Build history of the part. All positions in model axes, mm. A direction names the side the tool comes from. Coordinates: 2 decimals unless noted, no trailing zeros. Loops run counter-clockwise (first coordinate to the right, second up) from the corner with the lowest first, then second, coordinate; pieces in that order, holes last.
Item 1: 3-axis set-ups, long thin cutter, end or side, ignore diameter. For faces 4 (the face through (3, 325, -28)), 5 (the face through (206, -5, -25)), 6 (the face through (3, 331, -25)), 7 (the face through (224, -5, -56)): which of +Z, -Z, +X, -X, +Y, -Y reach the whole face in a straight line?
Item 2: Mould opens along X. For faces 1 (the face through (3, -331, -25)), 2 (the face through (-206, -5, -25)), 3 (the face through (3, -325, -28)) say: released by +X, released by -X, zero draft, split by the parting line, or undercut.
Item 3: Flat gauge pins, fed straight in: pin 1 (25 mm diameter, centred on y = -57, z = -19.5, fed in from +X); pin 2 (15 mm diameter, centred on x = 37.5, z = -15, fed in from -Y); pin 3 (15 mm diameter, centred on y = 155.5, z = -23.5, fed in from -X). Where does each tip first touch, or does it go through?
Item 4: Cut at A-A (z = -41). List the corners of the cut face in (x, y), and give its area (3 significant figures).
Item 5: Drill centre lines: line 1 along Y through (x, z) = (-88, -45); line 2 along X through (y, z) = (-148.5, -13.5); line 3 along Y through (x, z) = (74.5, -51). Where is each one in solid material? Low to high.
Item 6: Cut at C-C (y = -205). List the corners of the cut face in (x, z), and give its area (3 significant figures).
Item 7: Cut at B-B (x = 146.5). List the corners of the cut face in (y, z).
Item 8: Cut at D-D (x = 224). List the corners of the cut face in (y, z).
from build123d import *

# Parameters (mm, degrees)
SKETCH054_W            = 400
SKETCH054_H            = 60
PAD003_DEPTH           = 325
SKETCH055_W            = 412
SKETCH055_H            = 50
PAD008_DEPTH           = 331
SKETCH056_W            = 512
SKETCH056_H            = 762
PAD009_DEPTH           = 6
CUT003_PLACEMENT_ANGLE = 180


with BuildPart() as body002:
    # Sketch054 → Pad003 (new body, symmetric)
    with BuildSketch(Plane.XZ):
        with Locations((0, 30)):
            Rectangle(SKETCH054_W, SKETCH054_H)
    extrude(amount=PAD003_DEPTH, both=True)


with BuildPart() as cut003:
    # Sketch055 → Pad008 (new body, symmetric)
    with BuildSketch(Plane.XZ):
        with Locations((0, 25)):
            Rectangle(SKETCH055_W, SKETCH055_H)
    extrude(amount=PAD008_DEPTH, both=True)

    # Sketch056 (on Face3 of Pad008) → Pad009 (join)
    with BuildSketch(Plane(origin=(0, 0, 50), x_dir=(-1, 0, 0), z_dir=(0, 0, 1))):
        Rectangle(SKETCH056_W, SKETCH056_H)
    extrude(amount=PAD009_DEPTH)

    # Cut003: cut Body002
    add(body002.part, mode=Mode.SUBTRACT)


with BuildPart() as cut003_1:
    # Cut003 placement: moved
    add(cut003.part.rotate(Axis((0, 0, 0), (0, 1, 0)), CUT003_PLACEMENT_ANGLE))


solid = cut003_1.part
Filled sheet:
1. face 4: +Z, -Z
1. face 5: +Z, +X, +Y, -Y
1. face 6: +Z, +X, -X, +Y
1. face 7: -Z, +X, -X, +Y, -Y
2. face 1: zero draft
2. face 2: released by -X
2. face 3: undercut
3. pin 1: stops at x = 206
3. pin 2: stops at y = -331
3. pin 3: stops at x = -206
4. outline: (-206, -331) - (206, -331) - (206, 331) - (-206, 331) - close; hole (-200, -325) - (200, -325) - (200, 325) - (-200, 325) - close
4. area: 12,700 mm2
5. line 1: y = -331 to -325, 325 to 331
5. line 2: x = -206 to -200, 200 to 206
5. line 3: y = -381 to -325, 325 to 381
6. outline: (-256, -56) - (-200, -56) - (-200, 0) - (-206, 0) - (-206, -50) - (-256, -50) - close; (200, -56) - (256, -56) - (256, -50) - (206, -50) - (206, 0) - (200, 0) - close
6. area: 1,270 mm2
7. outline: (-381, -56) - (-325, -56) - (-325, 0) - (-331, 0) - (-331, -50) - (-381, -50) - close; (325, -56) - (381, -56) - (381, -50) - (331, -50) - (331, 0) - (325, 0) - close
8. outline: (-381, -56) - (381, -56) - (381, -50) - (-381, -50) - close
